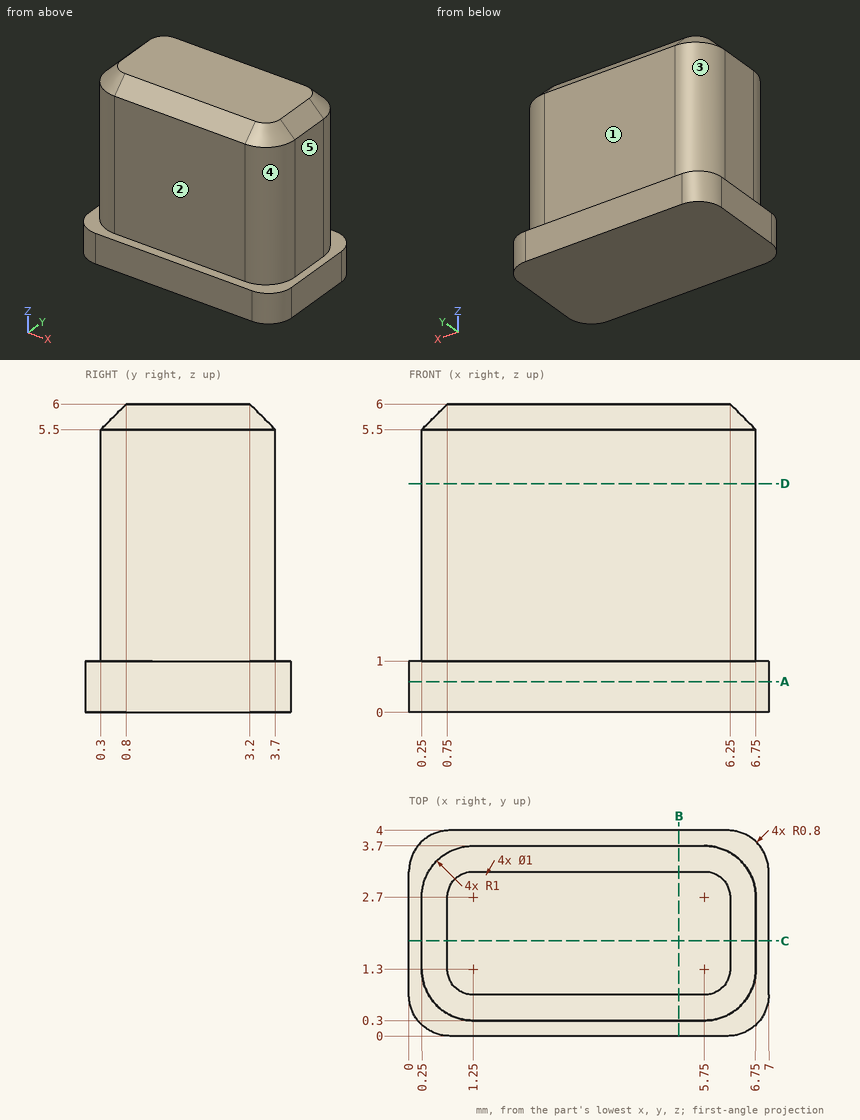
Geometry: see drawing. Coordinates: mm, zero at the bounding-box minimum. A direction names the side the tool comes from. Coordinates: 2 decimals unless noted, no trailing zeros. Order: outer loops, then holes, each group sorted by start corner. A loop starts at its lowest first (then second) coordinate and runs counter-clockwise, first axis right, second up. Notation, with made-up numbers: M 79.5,87.25 L 132.5,87.25 A23 cw 132.5,114.25 Z; hole C 7,-2.5 d5. An arc over 180 degrees is marked long. Write item = value, one per line. Start each with the question number.
(1) First-contact query: P1, Ø2, axis at x = 3.5, z = 3.5, coming from the +Y side; P2, Ø1.1, axis at y = 2, z = 3, coming from the -X side; P3, Ø2, axis at x = 3, z = 3, coming from the -Y side. Flat tips, straight axial feed; report the tip coordinate or a pass-through.
(2) Section C-C on y = 1.85. Output: boundary loops of the cut face in (x, z), and give its area (4 significant figures).
(3) Section D-D on z = 4.45. Output: boundary loops of the cut face in (x, y).
(4) Section A-A on z = 0.6. Output: boundary loops of the cut face in (x, y).
(5) Section B-B on x = 5.25. Output: boundary loops of the cut face in (y, z), and give its area (4 significant figures).
(6) Reachability of the marked faces 1, 2, 3, 4 and 5 from +Z, -Z, +X, -X, +Y, -Y: full face, straight path, thin tool, end or side. Return the list, or none.
(7) Line query: line 1 along Y through (x, z) = (1.5, 1.5); line 2 along X through (y, z) = (1.6, 3.35); line 3 along Z through (x, y) = (0.5, 3.5). Output: solid intervals per line, ascending. Write a range as [from, to].
Result set:
q1.P1 = 3.7
q1.P2 = 0.25
q1.P3 = 0.3
q2.outline = M 0,0 L 7,0 L 7,1 L 6.75,1 L 6.75,5.5 L 6.25,6 L 0.75,6 L 0.25,5.5 L 0.25,1 L 0,1 Z
q2.area = 39.25 mm²
q3.outline = M 0.25,1.3 A1 ccw 1.25,0.3 L 5.75,0.3 A1 ccw 6.75,1.3 L 6.75,2.7 A1 ccw 5.75,3.7 L 1.25,3.7 A1 ccw 0.25,2.7 Z
q4.outline = M 0,0.8 A0.8 ccw 0.8,0 L 6.2,0 A0.8 ccw 7,0.8 L 7,3.2 A0.8 ccw 6.2,4 L 0.8,4 A0.8 ccw 0,3.2 Z
q5.outline = M 0,0 L 4,0 L 4,1 L 3.7,1 L 3.7,5.5 L 3.2,6 L 0.8,6 L 0.3,5.5 L 0.3,1 L 0,1 Z
q5.area = 20.75 mm²
q6.face_1 = +Z, +X, -X, +Y
q6.face_2 = +Z, +X, -X, -Y
q6.face_3 = +Z, -X, +Y
q6.face_4 = +Z, +X, -Y
q6.face_5 = +Z, +X, +Y, -Y
q7.line_1 = [0.3, 3.7]
q7.line_2 = [0.25, 6.75]
q7.line_3 = [0, 1]
